from build123d import *

# Parameters (mm, degrees)
SKETCH_1_R      = 2.15
EXTRUDE_1_DEPTH = 300


with BuildPart() as part:
    # Эскиз1 → Бобышка-Вытянуть1 (new body)
    with BuildSketch(Plane.XY):
        with BuildLine():
            Line((-10, -2.75), (-10, -9.5))
            ThreePointArc((-10, -9.5), (-9.853553391, -9.853553391), (-9.5, -10))
            Line((-9.5, -10), (-2.75, -10))
            ThreePointArc((-2.75, -10), (-2.573223305, -9.926776695), (-2.5, -9.75))
            Line((-2.5, -9.75), (-2.5, -8.75))
            ThreePointArc((-2.5, -8.75), (-2.573223305, -8.573223305), (-2.75, -8.5))
            Line((-2.75, -8.5), (-6.5, -8.5))
            ThreePointArc((-6.5, -8.5), (-6.676776695, -8.426776695), (-6.75, -8.25))
            Line((-6.75, -8.25), (-6.75, -7.914213562))
            ThreePointArc((-6.75, -7.914213562), (-6.730969883, -7.818542704), (-6.676776695, -7.737436867))
            Line((-6.676776695, -7.737436867), (-3.085786438, -4.146446609))
            ThreePointArc((-3.085786438, -4.146446609), (-2.923574763, -4.038060234), (-2.732233047, -4))
            Line((-2.732233047, -4), (2.732233047, -4))
            ThreePointArc((2.732233047, -4), (2.923574763, -4.038060234), (3.085786438, -4.146446609))
            Line((3.085786438, -4.146446609), (6.676776695, -7.737436867))
            ThreePointArc((6.676776695, -7.737436867), (6.730969883, -7.818542704), (6.75, -7.914213562))
            Line((6.75, -7.914213562), (6.75, -8.25))
            ThreePointArc((6.75, -8.25), (6.676776695, -8.426776695), (6.5, -8.5))
            Line((6.5, -8.5), (2.75, -8.5))
            ThreePointArc((2.75, -8.5), (2.573223305, -8.573223305), (2.5, -8.75))
            Line((2.5, -8.75), (2.5, -9.75))
            ThreePointArc((2.5, -9.75), (2.573223305, -9.926776695), (2.75, -10))
            Line((2.75, -10), (9.5, -10))
            ThreePointArc((9.5, -10), (9.853553391, -9.853553391), (10, -9.5))
            Line((10, -9.5), (10, -2.75))
            ThreePointArc((10, -2.75), (9.926776695, -2.573223305), (9.75, -2.5))
            Line((9.75, -2.5), (8.75, -2.5))
            ThreePointArc((8.75, -2.5), (8.573223305, -2.573223305), (8.5, -2.75))
            Line((8.5, -2.75), (8.5, -6.5))
            ThreePointArc((8.5, -6.5), (8.426776695, -6.676776695), (8.25, -6.75))
            Line((8.25, -6.75), (7.914213562, -6.75))
            ThreePointArc((7.914213562, -6.75), (7.818542704, -6.730969883), (7.737436867, -6.676776695))
            Line((7.737436867, -6.676776695), (4.146446609, -3.085786438))
            ThreePointArc((4.146446609, -3.085786438), (4.038060234, -2.923574763), (4, -2.732233047))
            Line((4, -2.732233047), (4, 2.732233047))
            ThreePointArc((4, 2.732233047), (4.038060234, 2.923574763), (4.146446609, 3.085786438))
            Line((4.146446609, 3.085786438), (7.737436867, 6.676776695))
            ThreePointArc((7.737436867, 6.676776695), (7.818542704, 6.730969883), (7.914213562, 6.75))
            Line((7.914213562, 6.75), (8.25, 6.75))
            ThreePointArc((8.25, 6.75), (8.426776695, 6.676776695), (8.5, 6.5))
            Line((8.5, 6.5), (8.5, 2.75))
            ThreePointArc((8.5, 2.75), (8.573223305, 2.573223305), (8.75, 2.5))
            Line((8.75, 2.5), (9.75, 2.5))
            ThreePointArc((9.75, 2.5), (9.926776695, 2.573223305), (10, 2.75))
            Line((10, 2.75), (10, 9.5))
            ThreePointArc((10, 9.5), (9.853553391, 9.853553391), (9.5, 10))
            Line((9.5, 10), (2.75, 10))
            ThreePointArc((2.75, 10), (2.573223305, 9.926776695), (2.5, 9.75))
            Line((2.5, 9.75), (2.5, 8.75))
            ThreePointArc((2.5, 8.75), (2.573223305, 8.573223305), (2.75, 8.5))
            Line((2.75, 8.5), (6.5, 8.5))
            ThreePointArc((6.5, 8.5), (6.676776695, 8.426776695), (6.75, 8.25))
            Line((6.75, 8.25), (6.75, 7.810660172))
            Line((6.75, 7.810660172), (3.012563133, 4.073223305))
            ThreePointArc((3.012563133, 4.073223305), (2.931457296, 4.019030117), (2.835786438, 4))
            Line((2.835786438, 4), (-2.732233047, 4))
            ThreePointArc((-2.732233047, 4), (-2.923574763, 4.038060234), (-3.085786438, 4.146446609))
            Line((-3.085786438, 4.146446609), (-6.676776695, 7.737436867))
            ThreePointArc((-6.676776695, 7.737436867), (-6.730969883, 7.818542704), (-6.75, 7.914213562))
            Line((-6.75, 7.914213562), (-6.75, 8.25))
            ThreePointArc((-6.75, 8.25), (-6.676776695, 8.426776695), (-6.5, 8.5))
            Line((-6.5, 8.5), (-2.75, 8.5))
            ThreePointArc((-2.75, 8.5), (-2.573223305, 8.573223305), (-2.5, 8.75))
            Line((-2.5, 8.75), (-2.5, 9.75))
            ThreePointArc((-2.5, 9.75), (-2.573223305, 9.926776695), (-2.75, 10))
            Line((-2.75, 10), (-9.5, 10))
            ThreePointArc((-9.5, 10), (-9.853553391, 9.853553391), (-10, 9.5))
            Line((-10, 9.5), (-10, 2.75))
            ThreePointArc((-10, 2.75), (-9.926776695, 2.573223305), (-9.75, 2.5))
            Line((-9.75, 2.5), (-8.75, 2.5))
            ThreePointArc((-8.75, 2.5), (-8.573223305, 2.573223305), (-8.5, 2.75))
            Line((-8.5, 2.75), (-8.5, 6.5))
            ThreePointArc((-8.5, 6.5), (-8.426776695, 6.676776695), (-8.25, 6.75))
            Line((-8.25, 6.75), (-7.914213562, 6.75))
            ThreePointArc((-7.914213562, 6.75), (-7.818542704, 6.730969883), (-7.737436867, 6.676776695))
            Line((-7.737436867, 6.676776695), (-4.146446609, 3.085786438))
            ThreePointArc((-4.146446609, 3.085786438), (-4.038060234, 2.923574763), (-4, 2.732233047))
            Line((-4, 2.732233047), (-4, -2.732233047))
            ThreePointArc((-4, -2.732233047), (-4.038060234, -2.923574763), (-4.146446609, -3.085786438))
            Line((-4.146446609, -3.085786438), (-7.737436867, -6.676776695))
            ThreePointArc((-7.737436867, -6.676776695), (-7.818542704, -6.730969883), (-7.914213562, -6.75))
            Line((-7.914213562, -6.75), (-8.25, -6.75))
            ThreePointArc((-8.25, -6.75), (-8.426776695, -6.676776695), (-8.5, -6.5))
            Line((-8.5, -6.5), (-8.5, -2.75))
            ThreePointArc((-8.5, -2.75), (-8.573223305, -2.573223305), (-8.75, -2.5))
            Line((-8.75, -2.5), (-9.75, -2.5))
            ThreePointArc((-9.75, -2.5), (-9.926776695, -2.573223305), (-10, -2.75))
        make_face()
        with Locations(Location((0, 0, 0), (0, 0, 180))):
            Circle(SKETCH_1_R, mode=Mode.SUBTRACT)
    extrude(amount=-EXTRUDE_1_DEPTH)


solid = part.part
Input: part model. Units: mm. Frame: model coordinates. Give positions to 0.01 mm unless a question says otherwise; leave off trailing zeros.
Q1. Contact query for a flat-ended pin moving along its axis: pin 1 Ø2.5 at (y, z) = (0.5, -209.5) entering from +X. Output: stop coordinate, or through.
Checked values:
pin 1: stops at x = 4
Q2. Ray query, probe 1 along Y at (x, z) = (0, -117); probe 2 along X at (y, z) = (-8.75, -103.5); probe 3 along X at (y, z) = (-3, -162.5). Return the intervals inside material, ascending.
Checked values:
probe 1: y = -4 to -2.15, 2.15 to 4
probe 2: x = -10 to -2.5, 2.5 to 10
probe 3: x = -10 to -8.5, -4.08 to 4.08, 8.5 to 10
Q3. Draft query along Y for faces 1 (the flat face through (6, -10, -148)), 2 (the flat face through (-4, 0, -148)), 3 (the flat face through (10, -6, -148)). Return one class per face: +Y half, -Y half, draft (parallel to the pull), parting line (faces both ways), or undercut.
Checked values:
face 1: -Y half
face 2: undercut
face 3: draft
